```python
from build123d import *

# Parameters (mm, degrees)
SKETCH1_W                 = 419.1
SKETCH1_H                 = 311.15
SKETCH1_R                 = 116.5733
BOSS_EXTRUDE1_DEPTH       = 3.175
SKETCH2_R                 = 3.175
CUT_EXTRUDE1_DEPTH        = 3.175
CUT_EXTRUDE2_START        = -3.175
CUT_EXTRUDE2_DEPTH        = 3.175
SKETCH4_W                 = 107.95
SKETCH4_H                 = 3.175
SKETCH4_W_2               = 12.7
CUT_EXTRUDE3_DEPTH        = 3.175
MIRROR3_COPY_1_SKETCH_W   = 107.95
MIRROR3_COPY_1_SKETCH_H   = 3.175
MIRROR3_COPY_1_SKETCH_W_2 = 12.7
MIRROR3_COPY_1_DEPTH      = 3.175
SKETCH6_W                 = 6.35
SKETCH6_H                 = 50.8
SKETCH6_H_2               = 10.16
CUT_EXTRUDE4_DEPTH        = 3.175
MIRROR5_COPY_1_SKETCH_W   = 6.35
MIRROR5_COPY_1_SKETCH_H   = 50.8
MIRROR5_COPY_1_SKETCH_H_2 = 10.16
MIRROR5_COPY_1_DEPTH      = 3.175


with BuildPart() as part:
    # Sketch1 → Boss-Extrude1 (new body)
    with BuildSketch(Plane.XY):
        Rectangle(SKETCH1_W, SKETCH1_H)
        Circle(SKETCH1_R, mode=Mode.SUBTRACT)
        with BuildLine():
            Line((-86.296850441, 127), (-171.45, 127))
            ThreePointArc((-171.45, 127), (-175.940128061, 125.140128061), (-177.8, 120.65))
            Line((-177.8, 120.65), (-177.8, 19.05))
            ThreePointArc((-177.8, 19.05), (-175.940128061, 14.559871939), (-171.45, 12.7))
            Line((-171.45, 12.7), (-147.107669399, 12.7))
            ThreePointArc((-147.107669399, 12.7), (-142.915766684, 14.28025665), (-140.810252045, 18.234503425))
            ThreePointArc((-140.810252045, 18.234503425), (-121.830839941, 72.91961763), (-82.602635953, 115.485188356))
            ThreePointArc((-82.602635953, 115.485188356), (-80.250402974, 122.589838403), (-86.296850441, 127))
        make_face(mode=Mode.SUBTRACT)
        with BuildLine():
            Line((-177.8, -120.65), (-177.8, -19.05))
            ThreePointArc((-177.8, -19.05), (-175.940128061, -14.559871939), (-171.45, -12.7))
            Line((-171.45, -12.7), (-147.107669399, -12.7))
            ThreePointArc((-147.107669399, -12.7), (-142.915766684, -14.28025665), (-140.810252045, -18.234503425))
            ThreePointArc((-140.810252045, -18.234503425), (-121.830839941, -72.91961763), (-82.602635953, -115.485188356))
            ThreePointArc((-82.602635953, -115.485188356), (-80.250402974, -122.589838403), (-86.296850441, -127))
            Line((-86.296850441, -127), (-171.45, -127))
            ThreePointArc((-171.45, -127), (-175.940128061, -125.140128061), (-177.8, -120.65))
        make_face(mode=Mode.SUBTRACT)
        with BuildLine():
            Line((86.296850441, -127), (171.45, -127))
            ThreePointArc((171.45, -127), (175.940128061, -125.140128061), (177.8, -120.65))
            Line((177.8, -120.65), (177.8, -19.05))
            ThreePointArc((177.8, -19.05), (175.940128061, -14.559871939), (171.45, -12.7))
            Line((171.45, -12.7), (147.107669399, -12.7))
            ThreePointArc((147.107669399, -12.7), (142.915766684, -14.28025665), (140.810252045, -18.234503425))
            ThreePointArc((140.810252045, -18.234503425), (121.830839941, -72.91961763), (82.602635953, -115.485188356))
            ThreePointArc((82.602635953, -115.485188356), (80.250402974, -122.589838403), (86.296850441, -127))
        make_face(mode=Mode.SUBTRACT)
        with BuildLine():
            Line((177.8, 120.65), (177.8, 19.05))
            ThreePointArc((177.8, 19.05), (175.940128061, 14.559871939), (171.45, 12.7))
            Line((171.45, 12.7), (147.107669399, 12.7))
            ThreePointArc((147.107669399, 12.7), (142.915766684, 14.28025665), (140.810252045, 18.234503425))
            ThreePointArc((140.810252045, 18.234503425), (121.830839941, 72.91961763), (82.602635953, 115.485188356))
            ThreePointArc((82.602635953, 115.485188356), (80.250402974, 122.589838403), (86.296850441, 127))
            Line((86.296850441, 127), (171.45, 127))
            ThreePointArc((171.45, 127), (175.940128061, 125.140128061), (177.8, 120.65))
        make_face(mode=Mode.SUBTRACT)
    extrude(amount=BOSS_EXTRUDE1_DEPTH)

    # Sketch2 → Cut-Extrude1 (cut)
    with BuildSketch(Plane.XY.offset(3.175)):
        with Locations(Location((0, 122.936, 0), (0, 0, 180))):
            Circle(SKETCH2_R)
        with Locations((0, -122.936)):
            Circle(SKETCH2_R)
    extrude(amount=-CUT_EXTRUDE1_DEPTH, mode=Mode.SUBTRACT)

    # Sketch3 → Cut-Extrude2 (cut)
    with BuildSketch(Plane.XY.offset(3.175).offset(CUT_EXTRUDE2_START)):
        with BuildLine():
            Line((116.183512806, -9.525), (130.153512806, -9.525))
            ThreePointArc((130.153512806, -9.525), (133.745615254, -8.037102448), (135.233512806, -4.445))
            Line((135.233512806, -4.445), (135.233512806, 4.445))
            ThreePointArc((135.233512806, 4.445), (133.745615254, 8.037102448), (130.153512806, 9.525))
            Line((130.153512806, 9.525), (116.183512806, 9.525))
            ThreePointArc((116.183512806, 9.525), (116.5733, 0), (116.183512806, -9.525))
        make_face()
    cut_extrude2 = extrude(amount=CUT_EXTRUDE2_DEPTH, mode=Mode.SUBTRACT)

    # Mirror6: Cut-Extrude2 across plane
    add(cut_extrude2.mirror(Plane(origin=(0, 0, 0), x_dir=(0, 0, 1), z_dir=(1, 0, 0))), mode=Mode.SUBTRACT)

    # Sketch4 → Cut-Extrude3 (cut)
    with BuildSketch(Plane.XY.offset(3.175)):
        with Locations((-85.725, 153.9875)):
            Rectangle(SKETCH4_W, SKETCH4_H)
        with Locations((-184.15, 153.9875)):
            Rectangle(SKETCH4_W_2, SKETCH4_H)
        with Locations((-209.55, 153.9875)):
            Rectangle(SKETCH4_W_2, SKETCH4_H)
        with Locations((-158.75, 153.9875)):
            Rectangle(SKETCH4_W_2, SKETCH4_H)
    cut_extrude3 = extrude(amount=-CUT_EXTRUDE3_DEPTH, mode=Mode.SUBTRACT)

    # Mirror2: Cut-Extrude3 across plane
    add(cut_extrude3.mirror(Plane(origin=(0, 0, 0), x_dir=(0, 0, 1), z_dir=(1, 0, 0))), mode=Mode.SUBTRACT)

    # Mirror3: Cut-Extrude3 across plane
    add(cut_extrude3.mirror(Plane.ZX), mode=Mode.SUBTRACT)

    # Mirror3 copy 1 sketch → Mirror3 copy 1 (cut)
    with BuildSketch(Plane(origin=(0, 0, 3.175), x_dir=(-1, 0, 0), z_dir=(0, 0, 1))):
        with Locations((-85.725, 153.9875)):
            Rectangle(MIRROR3_COPY_1_SKETCH_W, MIRROR3_COPY_1_SKETCH_H)
        with Locations((-184.15, 153.9875)):
            Rectangle(MIRROR3_COPY_1_SKETCH_W_2, MIRROR3_COPY_1_SKETCH_H)
        with Locations((-209.55, 153.9875)):
            Rectangle(MIRROR3_COPY_1_SKETCH_W_2, MIRROR3_COPY_1_SKETCH_H)
        with Locations((-158.75, 153.9875)):
            Rectangle(MIRROR3_COPY_1_SKETCH_W_2, MIRROR3_COPY_1_SKETCH_H)
    extrude(amount=-MIRROR3_COPY_1_DEPTH, mode=Mode.SUBTRACT)

    # Sketch6 → Cut-Extrude4 (cut)
    with BuildSketch(Plane.XY.offset(3.175)):
        with Locations((-206.375, 127)):
            Rectangle(SKETCH6_W, SKETCH6_H)
        with Locations((-206.375, 25.4)):
            Rectangle(SKETCH6_W, SKETCH6_H)
        with Locations((-206.375, 86.36)):
            Rectangle(SKETCH6_W, SKETCH6_H_2)
        with Locations((-206.375, 66.04)):
            Rectangle(SKETCH6_W, SKETCH6_H_2)
    cut_extrude4 = extrude(amount=-CUT_EXTRUDE4_DEPTH, mode=Mode.SUBTRACT)

    # Mirror4: Cut-Extrude4 across plane
    add(cut_extrude4.mirror(Plane(origin=(0, 0, 0), x_dir=(0, 0, 1), z_dir=(1, 0, 0))), mode=Mode.SUBTRACT)

    # Mirror5: Cut-Extrude4 across plane
    add(cut_extrude4.mirror(Plane.ZX), mode=Mode.SUBTRACT)

    # Mirror5 copy 1 sketch → Mirror5 copy 1 (cut)
    with BuildSketch(Plane(origin=(0, 0, 3.175), x_dir=(-1, 0, 0), z_dir=(0, 0, 1))):
        with Locations((-206.375, 127)):
            Rectangle(MIRROR5_COPY_1_SKETCH_W, MIRROR5_COPY_1_SKETCH_H)
        with Locations((-206.375, 25.4)):
            Rectangle(MIRROR5_COPY_1_SKETCH_W, MIRROR5_COPY_1_SKETCH_H)
        with Locations((-206.375, 86.36)):
            Rectangle(MIRROR5_COPY_1_SKETCH_W, MIRROR5_COPY_1_SKETCH_H_2)
        with Locations((-206.375, 66.04)):
            Rectangle(MIRROR5_COPY_1_SKETCH_W, MIRROR5_COPY_1_SKETCH_H_2)
    extrude(amount=-MIRROR5_COPY_1_DEPTH, mode=Mode.SUBTRACT)


solid = part.part
```
Model file for the job. Use its own axes, mm. A direction names the side the tool comes from. Coordinates: 2 decimals unless noted, no trailing zeros. Loops run counter-clockwise (first coordinate to the right, second up) from the corner with the lowest first, then second, coordinate; pieces in that order, holes last. Notation, with made-up numbers: M 3,63 L 39,63 A24 cw 39,86 Z; hole C 41.25,-1.75 d10. An arc over 180 degrees is marked long. Use CSV: the item, a comma, the result in double quotes. Start each with the question number.
1. Band-saw the part on D-D, the plane z = 2.15. Give the number of separate pieces and of enclosed holes in the cut face, then the cut area to 3 significant figures.
2. Band-saw the part on A-A, the plane x = 65.5. List the corners of the cut face in (y, z) (3 decimals).
3. Flat gauge pins, fed straight in: pin 1 (1 mm diameter, centred on y = 153.5, z = 1.5, fed in from -X); pin 2 (1 mm diameter, centred on x = 156.5, z = 2, fed in from -Y); pin 3 (1 mm diameter, centred on x = -206, z = 1.5, fed in from +Y). Where does each tip first touch, or does it go through?
4. Band-saw the part on B-B, the plane x = -112. List the corners of the cut face in (y, z) (3 decimals), then the cut area to 3 significant figures.
5. Probe probe 1 along Y at (x, z) = (0, 1.8) (3 decimals); probe 2 along X at (y, z) = (-22, 1.75); probe 3 along X at (y, z) = (-31.5, 1.3). List the from-to ranges inside material, lowest first. Write a range as [from, to].
6. Band-saw the part on C-C, the plane y = -133. List the corners of the cut face in (x, z) (3 decimals), then the cut area to 3 significant figures.
7. Tool access for faces 1 (the cylindrical face through (2.43, 116.548, 1.565)), 2 (the flat face through (-50, 106, 0)): list every direction of +Z, -Z, +X, -X, +Y, -Y with a clear straight run to the whole face (end or side of a thin tool).
8. Two-plate mould, pull along X, no slides. Class faces 3 (the cylindrical face through (-122.248, 72.218, 1.565)), 4 (the flat face through (-50, 106, 3.175)): pulls with the +X half, pulls with the -X half, needs draft (parallel to the pull), parting line crosses it, or undercut.
Entries:
1,separate pieces,"1"
1,enclosed holes,"7"
1,area,"54,800 mm2"
2,outline,"M -152.4,0 L -96.432,0 L -96.432,3.175 L -152.4,3.175 Z; M 96.432,0 L 152.4,0 L 152.4,3.175 L 96.432,3.175 Z"
3,pin 1,"stops at x = -203.2"
3,pin 2,"stops at y = -152.4"
3,pin 3,"stops at y = 101.6"
4,outline,"M -152.4,0 L -127,0 L -127,3.175 L -152.4,3.175 Z; M -87.27,0 L -32.332,0 L -32.332,3.175 L -87.27,3.175 Z; M 32.332,0 L 87.27,0 L 87.27,3.175 L 32.332,3.175 Z; M 127,0 L 152.4,0 L 152.4,3.175 L 127,3.175 Z"
4,area,"510 mm2"
5,probe 1,"y = [-155.575, -126.111], [-119.761, -116.573], [116.573, 119.761], [126.111, 155.575]"
5,probe 2,"x = [-203.2, -177.8], [-140.27, -114.48], [114.48, 140.27], [177.8, 203.2]"
5,probe 3,"x = [-203.2, -177.8], [-138.45, -112.24], [112.24, 138.45], [177.8, 203.2]"
6,outline,"M -203.2,0 L 203.2,0 L 203.2,3.175 L -203.2,3.175 Z"
6,area,"1,290 mm2"
7,face 1,"+Z, -Z"
7,face 2,"-Z, +X, -X, +Y, -Y"
8,face 3,"undercut"
8,face 4,"needs draft"
